Source: CAD feature listing. Evaluate the final solid. Frame: model axes, mm. Round coordinates to 2 decimals unless told otherwise and drop trailing zeros. Order: outer loops, then holes, each group sorted by start corner. A loop starts at its lowest first (then second) coordinate and runs counter-clockwise, first axis right, second up. Notation, with made-up numbers: (0, 27.25) -> (12, 27.25) arc R24 cw to (12, 65.25) -> close; hole circle Ø9 at (9.25, -31). An arc over 180 degrees is marked (long way). Answer as CSV lines item,"result". Start each with the question number.
(1) Line query: line 1 along Y through (x, z) = (-10.5, 0.8); line 2 along X through (y, z) = (-7, 0.4); line 3 along Y through (x, z) = (-36, 0.8). Output: solid intervals per line, ascending. Write a range as from..to.
(2) Contact query for a flat-ended pin moving along its axis: P1, Ø5, axis at x = -43, y = -1.5, coming from the +Z side. Output: stop coordinate, or through.
(3) Section query D-D (z = 0.8). Count the separate pieces of the cut face and the enclosed holes in it, plus the area to 3 significant figures.
(4) Section query A-A (y = -20). Output: boundary loops of the cut face in (x, z).
(5) Section query C-C (y = 4). Output: boundary loops of the cut face in (x, z), plus the area to 3 significant figures.
(6) Section query B-B (x = -43). Output: boundary loops of the cut face in (y, z).
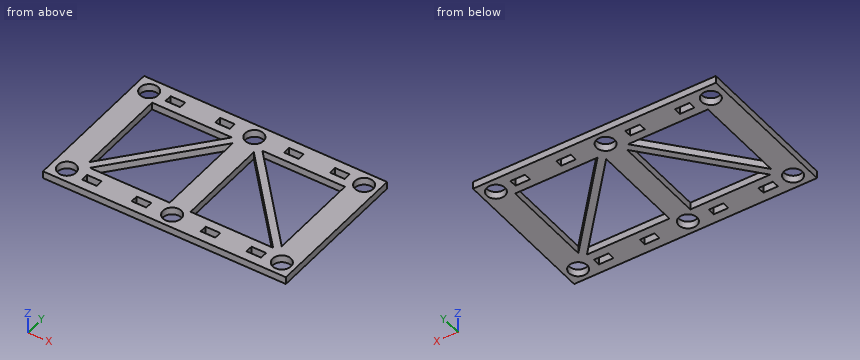
```python
from build123d import *

# Parameters (mm, degrees)
F0_W     = 66.5
F0_H     = 40.7
F0_R     = 2.5
F0_W_2   = 4
F0_H_2   = 2
F0_W_3   = 23.1688134372
F0_H_3   = 26.9576453138
F0_W_4   = 23.9260006735
F1_DEPTH = 2
F0_H_4   = 1.6511697322
F0_H_5   = 1.6511703735
F2_E4_W  = 35.5458655395
F2_E4_H  = 2
F3_DEPTH = 1
F4_E5_W  = 36.0439752121
F4_E5_H  = 2
F5_DEPTH = 1


with BuildPart() as f1:
    # F0 (on Top) → F1 (new body)
    with BuildSketch(Plane.XY):
        with Locations((-26.3848016039, -10.9677366539)):
            Rectangle(F0_W, F0_H)
        with Locations((-55.6704513729, -27.5134705007)):
            Circle(F0_R, mode=Mode.SUBTRACT)
        with Locations((-48.6798131391, -27.7539507372)):
            Rectangle(F0_W_2, F0_H_2, mode=Mode.SUBTRACT)
        with Locations((-35.1007831245, -27.7539507372)):
            Rectangle(F0_W_2, F0_H_2, mode=Mode.SUBTRACT)
        with Locations((-26.8697291613, -27.5134705007)):
            Circle(F0_R, mode=Mode.SUBTRACT)
        with Locations((-16.2120581007, -27.7539507372)):
            Rectangle(F0_W_2, F0_H_2, mode=Mode.SUBTRACT)
        with Locations((-3.6603234261, -27.7539507372)):
            Rectangle(F0_W_2, F0_H_2, mode=Mode.SUBTRACT)
        with Locations((3.1705482397, -27.5134705007)):
            Circle(F0_R, mode=Mode.SUBTRACT)
        with Locations((-55.6704513729, 5.5923270993)):
            Circle(F0_R, mode=Mode.SUBTRACT)
        with Locations((-48.6798131391, 5.8541836441)):
            Rectangle(F0_W_2, F0_H_2, mode=Mode.SUBTRACT)
        with Locations((-41.2725005299, -10.8643159037)):
            Rectangle(F0_W_3, F0_H_3, mode=Mode.SUBTRACT)
        with Locations((-35.1007831245, 5.8541836441)):
            Rectangle(F0_W_2, F0_H_2, mode=Mode.SUBTRACT)
        with Locations((-26.8697291613, 5.5923270993)):
            Circle(F0_R, mode=Mode.SUBTRACT)
        with Locations((-12.0121349685, -10.8643159037)):
            Rectangle(F0_W_4, F0_H_3, mode=Mode.SUBTRACT)
        with Locations((-16.2120581007, 5.8541836441)):
            Rectangle(F0_W_2, F0_H_2, mode=Mode.SUBTRACT)
        with Locations((-3.6603234261, 5.8541836441)):
            Rectangle(F0_W_2, F0_H_2, mode=Mode.SUBTRACT)
        with Locations((3.1705482397, 5.5923270993)):
            Circle(F0_R, mode=Mode.SUBTRACT)
    extrude(amount=F1_DEPTH)

    # F2_E4 (on explicit) → F3 (join, symmetric)
    with BuildSketch(Plane(origin=(-52.8569072485, -24.3431385607, 0), x_dir=(0.6518005142, 0.7583904599, 0), z_dir=(0.7583904599, -0.6518005142, 0))):
        with Locations((17.7729327698, 1)):
            Rectangle(F2_E4_W, F2_E4_H)
    extrude(amount=F3_DEPTH, both=True)

    # F4_E5 (on explicit) → F5 (join, symmetric)
    with BuildSketch(Plane(origin=(-23.9751353052, 2.6145067532, 0), x_dir=(0.6638002754, -0.7479098838, 0), z_dir=(-0.7479098838, -0.6638002754, 0))):
        with Locations((18.0219876061, 1)):
            Rectangle(F4_E5_W, F4_E5_H)
    extrude(amount=F5_DEPTH, both=True)


with BuildPart() as f1b:
    # F0 (on Top) → F1, piece 2 (new body)
    with BuildSketch(Plane.XY):
        with Locations((-3.6603234261, 39.867881812)):
            Rectangle(F0_W_2, F0_H_4)
    extrude(amount=F1_DEPTH)


with BuildPart() as f1c:
    # F0 (on Top) → F1, piece 3 (new body)
    with BuildSketch(Plane.XY):
        with Locations((-3.6603234261, -61.797210648)):
            Rectangle(F0_W_2, F0_H_5)
    extrude(amount=F1_DEPTH)


solid = f1.part
```
Answer block:
1,line 1,"-31.32..-24.34, -14.07..-11.06, 2.61..9.38"
1,line 2,"-59.63..-52.86, -39.27..-36.63, -29.69..-23.98, -16.78..-14.1, -0.05..6.87"
1,line 3,"-31.32..-28.75, -26.75..-24.34, -6.26..-3.2, 2.61..4.85, 6.85..9.38"
2,P1,"through"
3,separate pieces,"1"
3,enclosed holes,"18"
3,area,"1,390 mm2"
4,outline,"(-59.63, 0) -> (-52.86, 0) -> (-52.86, 2) -> (-59.63, 2) -> close; (-50.44, 0) -> (-47.81, 0) -> (-47.81, 2) -> (-50.44, 2) -> close; (-29.69, 0) -> (-23.98, 0) -> (-23.98, 2) -> (-29.69, 2) -> close; (-5.24, 0) -> (-2.57, 0) -> (-2.57, 2) -> (-5.24, 2) -> close; (-0.05, 0) -> (6.87, 0) -> (6.87, 2) -> (-0.05, 2) -> close"
5,outline,"(-59.63, 0) -> (-57.6, 0) -> (-57.6, 2) -> (-59.63, 2) -> close; (-53.74, 0) -> (-28.8, 0) -> (-28.8, 2) -> (-53.74, 2) -> close; (-24.94, 0) -> (1.24, 0) -> (1.24, 2) -> (-24.94, 2) -> close; (5.1, 0) -> (6.87, 0) -> (6.87, 2) -> (5.1, 2) -> close"
5,area,"110 mm2"
6,outline,"(-31.32, 0) -> (-24.34, 0) -> (-24.34, 2) -> (-31.32, 2) -> close; (-14.41, 0) -> (-11.34, 0) -> (-11.34, 2) -> (-14.41, 2) -> close; (2.61, 0) -> (9.38, 0) -> (9.38, 2) -> (2.61, 2) -> close"
